Source: three-view drawing plus pictorial views. Frame: mm from the lowest corner of the part. A direction names the side the tool comes from. Coordinates: 2 decimals unless noted, no trailing zeros. Order: outer loops, then holes, each group sorted by start corner. A loop starts at its lowest first (then second) coordinate and runs counter-clockwise, first axis right, second up. Notation, with made-up numbers: M -36.5,14 L -18.5,14 A19 ccw -18.5,43 Z; hole C 68.5,89 d4. An arc over 180 degrees is marked long. One line per question, with ' | ' between items.
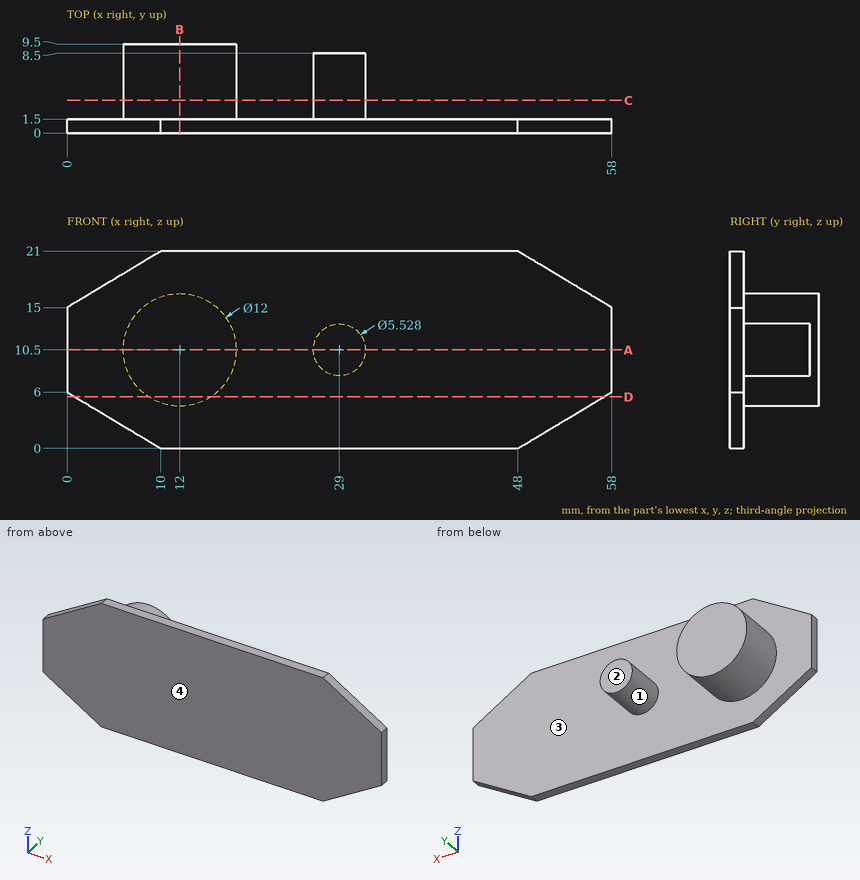
1. Section D-D, the plane z = 5.5. Output: boundary loops of the cut face in (x, y).
Response values:
outline: M 0.83,0 L 57.17,0 L 57.17,1.5 L 15.32,1.5 L 15.32,9.5 L 8.68,9.5 L 8.68,1.5 L 0.83,1.5 Z
2. Section B-B, the plane x = 12. Output: boundary loops of the cut face in (y, z).
Response values:
outline: M 0,0 L 1.5,0 L 1.5,4.5 L 9.5,4.5 L 9.5,16.5 L 1.5,16.5 L 1.5,21 L 0,21 Z
3. Draft query along X for the marked faces 1 and 2. Return one class per face: pulls with the +X half, pulls with the -X half, needs draft (parallel to the pull), parting line crosses it, or undercut.
Response values:
face 1: undercut | face 2: needs draft
4. Pin query (flat end, axial travel): P1, Ø5, axis at x = 15.5, z = 5.5, coming from the +Y side; P2, Ø2, axis at y = 6, z = 16.5, coming from the -X side; P3, Ø1.7, axis at x = 28, z = 11.5, coming from the +Y side; P4, Ø3, axis at x = 11.5, y = 7.5, coming from the +Z side. Return the tip coordinate at first contact, or that it passes through.
Response values:
P1: stops at y = 9.5 | P2: stops at x = 8.68 | P3: stops at y = 8.5 | P4: stops at z = 16.5
5. Section C-C, the plane y = 3.5. Output: boundary loops of the cut face in (x, z).
Response values:
outline: C 12,10.5 d12; C 29,10.5 d5.53
6. Material intervals for line 1 (Y direction, x = 19, z = 12.5); line 2 (X direction, y = 2.5, z = 12.75) (1 decimal); line 3 (X direction, y = 8, z = 11.5), sorted ascending. Write a range as [from, to].
Response values:
line 1: y = [0, 1.5] | line 2: x = [6.4, 17.6], [27.4, 30.6] | line 3: x = [6.08, 17.92], [26.42, 31.58]
7. Section A-A, the plane z = 10.5. Output: boundary loops of the cut face in (x, y).
Response values:
outline: M 0,0 L 58,0 L 58,1.5 L 31.76,1.5 L 31.76,8.5 L 26.24,8.5 L 26.24,1.5 L 18,1.5 L 18,9.5 L 6,9.5 L 6,1.5 L 0,1.5 Z
8. Access query for the marked faces 3 and 4. Directions: +Z, -Z, +X, -X, +Y, -Y. A direction counts if a zero-diameter tool reaches every point of the face in a straight line with its end or side. Return the directions, or none.
Response values:
face 3: +Y | face 4: +Z, -Z, +X, -X, -Y
